Here's how the part is built. I have some questions about the finished solid (model axes, mm). A direction names the side the tool comes from. Round coordinates to 2 decimals unless told otherwise and drop trailing zeros. Write each loop counter-clockwise with the first axis right and the second up, starting at its lowest first coordinate (ties: lowest second). Pieces come first, ordered by that corner, then holes. Notation, with made-up numbers: (86, -35) -> (108, -35) arc R35 ccw to (108, 0) -> close; hole circle Ø6 at (79, 87). An arc over 180 degrees is marked (long way). Put each result on its own line as item: value. Start each with the question number.
1) We'd pull the mould along Z, two halves only. Please class faces 1 (the flat face through (58, 6.5, -40)), 2 (the flat face through (86.049, 24.65, -51.412)), 3 (the flat face through (98.205, 22.876, 17.316)): released by +Z, released by -Z, zero draft, split by the parting line, or undercut.
2) I want a section at C-C, the plane x = 85. List the corners of the cut face in (y, z) for me.
3) I want a section at A-A, the plane x = 20.5. List the corners of the cut face in (y, z) for me, then the cut area to 3 significant figures.
4) Which directions (+Z, -Z, +X, -X, +Y, -Y) give clear straight access to the entire face, cutting with the end or side of a thin tool? Please do faces 4 (the flat face through (58, -3.5, -64)), 5 (the cylindrical face through (41.34, 24.65, -71.97)).
5) If I drill on line 1 along Z through (x, y) = (72.5, 41.5); line 2 along X through (y, z) = (47.5, -65.5); line 3 along Z through (x, y) = (70.5, 24.5), over which ranges is the centre line in solid material (lowest first)? Write a range as [from, to].
6) Will these pins go through, and if not, where does the flat tip stop? P1, Ø22, axis at x = 49.5, z = -88.5, coming from the +Y side; P2, Ø6, axis at y = 18.5, z = -48, coming from the -X side; P3, Ø1, axis at y = 16.5, z = -64, coming from the +X side.
7) I want a section at B-B, the plane y = 23. List the corners of the cut face in (x, z) for me.
8) I want a section at D-D, the plane z = -48.5. List the corners of the cut face in (x, y) for me, then the cut area to 3 significant figures.
Autodesk Inventor part; units mm, degrees
ref_plane "Plan de construction1" through (0, 0, 0) normal (0.766, 0, 0.6428) x (0.6422, -0.0437, -0.7653)
ref_plane "YZ Plane" through (0, 0, 0) normal (1, 0, 0) x (0, 1, 0)
ref_plane "XZ Plane" through (0, 0, 0) normal (0, 1, 0) x (-1, 0, 0)
sketch "Esquisse1" plane through (0, 0, 0) normal (0, 1, 0) x (-1, 0, 0)
  circle A0 centre (0, 0) radius 100
  line L0 (0, 0) -> (-118.1769, 20.8378)
  line L1 (0, 0) -> (-2.1593, 0)
  line L2 (0, 0) -> (-118.1769, -20.8378)
  arc A1 (-118.1769, 20.8378) -> (-118.1769, -20.8378) centre (0, 0) ccw
  line L3 (-118.1769, 20.8378) -> (-78.7846, 13.8919)
  arc A2 (-78.7846, 13.8919) -> (-78.7846, -13.8919) centre (0, 0) ccw
  line L4 (-78.7846, -13.8919) -> (-118.1769, -20.8378)
  arc A3 (-115.2225, 20.3168) -> (-115.2225, -20.3168) centre (0, 0) ccw
  arc A4 (-81.739, 14.4128) -> (-81.739, -14.4128) centre (0, 0) ccw
  line L5 (-115.4735, 18.838) -> (-81.9862, 12.9332)
  line L6 (-115.4735, -18.838) -> (-81.9862, -12.9332)
  dimension "d0" = 200
  dimension "d1" = 10
  dimension "d2" = 10
  dimension "d3" = 40
  dimension "d4" = 120
  dimension "d5" = 117
  dimension "d6" = 83
  dimension "d7" = 1.5
  dimension "d8" = 1.5
extrude "Extrusion2" add sketch "Esquisse1" along normal blind 50 and the other way blind 3.5 contours L0 A4 L5 A0 | A0 L5 A3 L0 | L2 A3 L6 A0 | A0 L6 A4 L2 | L5 A4 L6 A0 | A0 L6 A3 L5 | L0 A2 L2 A4 | A3 L2 A1 L0
extrude "Extrusion3" cut sketch "Esquisse1" along normal blind 60 contours L5 A4 L6 A0 | A0 L6 A3 L5
pattern_circular "Réseau circulaire1" count 6 over 100 about axis through (0, -10, 0) along (0, 1, 0) of "Extrusion2", "Extrusion3"
sketch "Esquisse2" plane through (0, -3.5, 0) normal (0, -1, 0) x (1, 0, 0)
  line L0 (0, 0) -> (51.423, -61.2836)
  arc A0 (-27.3616, -75.1754) -> (78.7846, 13.8919) centre (0, 0) ccw
  line L1 (0, 0) -> (78.7846, 13.8919)
  line L2 (62.0017, -50.5549) -> (69.6621, -44.127)
  line L3 (69.6621, -44.127) -> (56.8064, -28.8061)
  line L4 (56.8064, -28.8061) -> (49.1459, -35.234)
  line L5 (49.1459, -35.234) -> (62.0017, -50.5549)
  dimension "d20" = 60
  dimension "d21" = 10
  dimension "d22" = 15
  dimension "d23" = 20
extrude "Extrusion4" add sketch "Esquisse2" against normal blind 10 contours L5 L4 L3 A0 | A0 L3 L2
ref_plane "Plan de construction1" through (0, 0, 0) normal (0.766, 0, 0.6428) x (0.6422, -0.0437, -0.7653)
mirror "Symétrie1" about plane through (0, 0, 0) normal (0.766, 0, 0.6428) of "Extrusion4"
properties part number "bacRecupBonbon"
Findings:
1. face 1: zero draft
1. face 2: undercut
1. face 3: released by +Z
2. outline: (-3.5, -84.71) -> (50, -84.71) -> (50, -80.4) -> (0, -80.4) -> (0, -50.81) -> (50, -50.81) -> (50, -47.34) -> (0, -47.34) -> (0, -16.51) -> (50, -16.51) -> (50, -13.46) -> (0, -13.46) -> (0, 13.46) -> (50, 13.46) -> (50, 14.99) -> (-3.5, 14.99) -> close
3. outline: (-3.5, -118.24) -> (50, -118.24) -> (50, -115.19) -> (0, -115.19) -> (0, -80.43) -> (50, -80.43) -> (50, -77.33) -> (-3.5, -77.33) -> close; (-3.5, -63.32) -> (6.5, -63.32) -> (6.5, -59.27) -> (-3.5, -59.27) -> close
3. area: 491 mm2
4. face 4: +Z, -Z, +X, -X, -Y
4. face 5: +Y
5. line 1: z = [-95.62, -91.83], [-88.74, -84.07], [-43.59, -33.82]
5. line 2: x = [45.93, 50.98], [53, 56.92], [96.95, 100.55]
5. line 3: z = [-97.11, -93.37], [-86.35, -81.69], [-43.8, -37.81]
6. P1: stops at y = 0
6. P2: stops at x = 61.64
6. P3: stops at x = 101.82
7. outline: (-41.04, -112.76) arc R120 ccw to (118.18, 20.84) -> (78.78, 13.89) arc R80 cw to (-27.36, -75.18) -> close; hole (-38.6, -110.45) arc R117 ccw to (-1.5, -116.99) -> (-1.5, -82.99) arc R83 cw to (-26.97, -78.49) -> close; hole (1.5, -116.99) arc R117 ccw to (38.6, -110.45) -> (26.97, -78.49) arc R83 cw to (1.5, -82.99) -> close; hole (29.79, -77.47) -> (41.42, -109.42) arc R117 ccw to (74.05, -90.58) -> (52.19, -64.54) arc R83 cw to start; hole (54.49, -62.61) -> (76.35, -88.66) arc R117 ccw to (100.57, -59.79) -> (71.12, -42.79) arc R83 cw to start; hole (72.62, -40.19) -> (102.07, -57.2) arc R117 ccw to (114.95, -21.79) -> (81.47, -15.89) arc R83 cw to start; hole (81.99, -12.93) -> (115.47, -18.84) arc R117 ccw to (115.47, 18.84) -> (81.99, 12.93) arc R83 cw to start
8. outline: (60.28, -3.5) -> (109.76, -3.5) -> (109.76, 50) -> (106.47, 50) -> (106.47, 0) -> (87, 0) -> (87, 50) -> (81, 50) -> (81, 0) -> (67.36, 0) -> (67.36, 50) -> (63.62, 50) -> (63.62, 6.5) -> (60.28, 6.5) -> close
8. area: 846 mm2
